```python
from build123d import *

# Parameters (mm, degrees)
SKETCH_1_R          = 1
EXTRUDE_1_DEPTH     = 1.6
SKETCH_2_W          = 16.76
SKETCH_2_H          = 9.2
EXTRUDE_2_DEPTH     = 15.2
CUT_EXTRUDE_START   = -15.2
SKETCH_3_W          = 12.83
SKETCH_3_H          = 1.6
CUT_EXTRUDE_2_DEPTH = 9
CUT_EXTRUDE_3_DEPTH = 15.2
EXTRUDE_START       = 1.6
SKETCH_7_W          = 3.6
SKETCH_7_H          = 15
EXTRUDE_4_DEPTH     = 4.5


with BuildPart() as part:
    # 草图1 → 凸台-拉伸1 (new body)
    with BuildSketch(Plane(origin=(0, 0, 0), x_dir=(1, 0, 0), z_dir=(0, 1, 0))):
        with BuildLine():
            Line((-10.65, 12.5), (10.65, 12.5))
            ThreePointArc((10.65, 12.5), (11.958147545, 11.958147545), (12.5, 10.65))
            Line((12.5, 10.65), (12.5, -10.65))
            ThreePointArc((12.5, -10.65), (11.958147545, -11.958147545), (10.65, -12.5))
            Line((10.65, -12.5), (-10.65, -12.5))
            ThreePointArc((-10.65, -12.5), (-11.958147545, -11.958147545), (-12.5, -10.65))
            Line((-12.5, -10.65), (-12.5, 10.65))
            ThreePointArc((-12.5, 10.65), (-11.958147545, 11.958147545), (-10.65, 12.5))
        make_face()
        with Locations(Location((-10.65, 10.65, 0), (0, 0, 270))):
            Circle(SKETCH_1_R, mode=Mode.SUBTRACT)
        with Locations(Location((-10.65, -10.65, 0), (0, 0, 270))):
            Circle(SKETCH_1_R, mode=Mode.SUBTRACT)
        with Locations(Location((10.65, -10.65, 0), (0, 0, 270))):
            Circle(SKETCH_1_R, mode=Mode.SUBTRACT)
        with Locations(Location((10.65, 10.65, 0), (0, 0, 270))):
            Circle(SKETCH_1_R, mode=Mode.SUBTRACT)
    extrude(amount=EXTRUDE_1_DEPTH)

    # 草图2 → 凸台-拉伸2 (add)
    with BuildSketch(Plane(origin=(0, 0, 0), x_dir=(1, 0, 0), z_dir=(0, 1, 0))):
        with Locations((0, 4.8)):
            Rectangle(SKETCH_2_W, SKETCH_2_H)
        with Locations((0, -4.8)):
            Rectangle(SKETCH_2_W, SKETCH_2_H)
    extrude(amount=-EXTRUDE_2_DEPTH)

    # 草图3 → 切除-拉伸2 (cut)
    with BuildSketch(Plane(origin=(0, 0, 0), x_dir=(1, 0, 0), z_dir=(0, 1, 0)).offset(CUT_EXTRUDE_START)):
        with Locations((0, -4.8)):
            Rectangle(SKETCH_3_W, SKETCH_3_H)
        with Locations((0, 4.8)):
            Rectangle(SKETCH_3_W, SKETCH_3_H)
    extrude(amount=CUT_EXTRUDE_2_DEPTH, mode=Mode.SUBTRACT)

    # 草图5 → 切除-拉伸3 (cut)
    with BuildSketch(Plane(origin=(0, 0, 0), x_dir=(1, 0, 0), z_dir=(0, 1, 0)).offset(CUT_EXTRUDE_START)):
        Polygon((-8.38, -9.4), (-8.38, -8.4), (-7.38, -9.4), align=None)
        Polygon((7.38, -9.4), (8.38, -9.4), (8.38, -8.4), align=None)
        Polygon((-8.38, -0.2), (-8.38, -1.2), (-7.38, -0.2), align=None)
        Polygon((8.38, -0.2), (7.38, -0.2), (8.38, -1.2), align=None)
        Polygon((-8.38, 0.2), (-7.38, 0.2), (-8.38, 1.2), align=None)
        Polygon((-8.38, 9.4), (-7.38, 9.4), (-8.38, 8.4), align=None)
        Polygon((8.38, 9.4), (7.38, 9.4), (8.38, 8.4), align=None)
        Polygon((7.38, 0.2), (8.38, 0.2), (8.38, 1.2), align=None)
    extrude(amount=CUT_EXTRUDE_3_DEPTH, mode=Mode.SUBTRACT)

    # 草图7 → 凸台-拉伸4 (add)
    with BuildSketch(Plane(origin=(0, 0, 0), x_dir=(1, 0, 0), z_dir=(0, 1, 0)).offset(EXTRUDE_START)):
        with Locations((-10.6, 0)):
            Rectangle(SKETCH_7_W, SKETCH_7_H)
    extrude(amount=EXTRUDE_4_DEPTH)


solid = part.part
```
For this review, take the finished solid that the model builds, in its own axes (mm). A direction names the side the tool comes from. Give positions to 0.01 mm unless a question says otherwise; leave off trailing zeros. Write each loop counter-clockwise with the first axis right and the second up, starting at its lowest first coordinate (ties: lowest second). Pieces come first, ordered by that corner, then holes. Notation, with made-up numbers: M 77.5,50.25 L 126.5,50.25 A20 cw 126.5,75.25 Z; hole C -17,5.5 d10. An arc over 180 degrees is marked long. One line per item, written item: value.
1) For P1, Ø4, axis at y = -4.5, z = 6, coming from the +X side; P2, Ø1.5, axis at x = 6.5, z = 6, coming from the +Y side; P3, Ø1.6, axis at x = -10.65, z = -10.65, coming from the +Y side; P4, Ø5, axis at x = 8, y = -11, coming from the +Z side, all flat-tipped, find the tip position at first contact; note any pin that passes through.
Results are:
P1: stops at x = 8.38
P2: stops at y = 1.6
P3: passes through
P4: stops at z = 9.4
2) Take a section at D-D, the plane x = 0.5. Write out the cut boundary in (y, z).
Results are:
outline: M -15.2,-9.4 L 0,-9.4 L 0,-12.5 L 1.6,-12.5 L 1.6,12.5 L 0,12.5 L 0,9.4 L -15.2,9.4 L -15.2,5.6 L -6.2,5.6 L -6.2,4 L -15.2,4 L -15.2,0.2 L 0,0.2 L 0,-0.2 L -15.2,-0.2 L -15.2,-4 L -6.2,-4 L -6.2,-5.6 L -15.2,-5.6 Z
3) The part is to be moulded in two halves that separate along X. For faces 5 (the flat face through (-0.1, -15.2, -3.8)), 6 (the flat face through (-6.415, -11, 5)), 7 (the cylindrical face through (-11.944, 0.789, 11.972)), say which applies: +X half, -X half, draft (parallel to the pull), parting line (faces both ways), or undercut.
Results are:
face 5: draft
face 6: undercut
face 7: -X half
4) Take a section at A-A, the plane y = -14. Write out the cut boundary in (x, z) (3 decimals), then the cut area to 3 significant figures.
Results are:
outline: M -8.38,-8.4 L -7.38,-9.4 L 7.38,-9.4 L 8.38,-8.4 L 8.38,-1.2 L 7.38,-0.2 L -7.38,-0.2 L -8.38,-1.2 Z; M -8.38,1.2 L -7.38,0.2 L 7.38,0.2 L 8.38,1.2 L 8.38,8.4 L 7.38,9.4 L -7.38,9.4 L -8.38,8.4 Z; hole M -6.415,-5.6 L 6.415,-5.6 L 6.415,-4 L -6.415,-4 Z; hole M -6.415,4 L 6.415,4 L 6.415,5.6 L -6.415,5.6 Z
area: 263 mm²
5) For line 1 (Z direction, x = -3.75, y = -11); line 2 (X direction, y = 1.05, z = 10.65); line 3 (X direction, y = -5, z = -1.25), list the stretches that pass through material, from the lowest coordinate up. Write a range as from..to.
Results are:
line 1: z = -9.4..-5.6, -4..-0.2, 0.2..4, 5.6..9.4
line 2: x = -12.5..-11.65, -9.65..9.65, 11.65..12.5
line 3: x = -8.38..8.38
6) Take a section at C-C, the plane z = -4.5. Write out the cut boundary in (x, y) (3 decimals).
Results are:
outline: M -12.5,0 L -8.38,0 L -8.38,-15.2 L -6.415,-15.2 L -6.415,-6.2 L 6.415,-6.2 L 6.415,-15.2 L 8.38,-15.2 L 8.38,0 L 12.5,0 L 12.5,1.6 L -8.8,1.6 L -8.8,6.1 L -12.4,6.1 L -12.4,1.6 L -12.5,1.6 Z
7) Take a section at B-B, the plane y = -1.25. Write out the cut boundary in (x, z).
Results are:
outline: M -8.38,-8.4 L -7.38,-9.4 L 7.38,-9.4 L 8.38,-8.4 L 8.38,-1.2 L 7.38,-0.2 L -7.38,-0.2 L -8.38,-1.2 Z; M -8.38,1.2 L -7.38,0.2 L 7.38,0.2 L 8.38,1.2 L 8.38,8.4 L 7.38,9.4 L -7.38,9.4 L -8.38,8.4 Z
8) For faces 1 (the flat face through (7.87, -7.71, 0.69)), 2 (the flat face through (0, -7, 9.4)), 3 (the flat face through (-7.87, -7.71, -8.91)), 4 (the flat face through (0, -7, 0.2)), list the 3-axis set-ups (+Z, -Z, +X, -X, +Y, -Y) from which the entire face can be reached by the end or side of a thin tool; tool diameter is ignored.
Results are:
face 1: +X, -Y
face 2: +Z, +X, -X, -Y
face 3: -Z, -X, -Y
face 4: +X, -X, -Y
